Geometry check sheet. Reference: the model listing, model coordinates, mm. Round coordinates to 2 decimals unless told otherwise and drop trailing zeros. Loops run counter-clockwise (first coordinate to the right, second up) from the corner with the lowest first, then second, coordinate; pieces in that order, holes last. Notation, with made-up numbers: M 69,29 L 118,29 A19 cw 118,58 Z; hole C -14,82 d10. An arc over 180 degrees is marked long. Answer in a Markdown table with one row per item. Add a question column.
```python
from build123d import *

# Parameters (mm, degrees)
SKETCH1_R               = 8.89
SKETCH1_R_2             = 6.35
BOSS_EXTRUDE1_DEPTH     = 12.7
CUT_EXTRUDE1_DEPTH      = 29.341210278
CUT_EXTRUDE1_DEPTH_BACK = 29.341210278
SKETCH4_W               = 12.7
SKETCH4_H               = 5.08


# Read off the part's stored shape, not the designer's step: Revolve6
with BuildPart() as part:
    # Sketch1 → Boss-Extrude1 (new body)
    with BuildSketch(Plane(origin=(0, 0, 0), x_dir=(1, 0, 0), z_dir=(0, 1, 0))):
        with Locations(Location((0, 0, 0), (0, 0, 270))):
            Circle(SKETCH1_R)
        with Locations(Location((0, 0, 0), (0, 0, 270))):
            Circle(SKETCH1_R_2, mode=Mode.SUBTRACT)
    extrude(amount=BOSS_EXTRUDE1_DEPTH)

    # Revolve6 outline → Revolve6 (revolve)
    with BuildSketch(Plane.XY):
        Polygon((6.35, 0), (5.309918247, -2.54), (0, -17.711194992), (0, -25.4), (8.89, 0), align=None)
    revolve(axis=Axis((0, 0, 0), (0, 1, 0)))

    # Sketch4 → Cut-Extrude1 (cut, two sides: drawn at the far end of the back side and taken through both)
    with BuildSketch(Plane.XY.offset(-CUT_EXTRUDE1_DEPTH_BACK)):
        with Locations((0, -24.13)):
            Rectangle(SKETCH4_W, SKETCH4_H)
    extrude(amount=CUT_EXTRUDE1_DEPTH + CUT_EXTRUDE1_DEPTH_BACK, mode=Mode.SUBTRACT)


solid = part.part
```
1) Cross-section at A-A, the plane y = 10. Record the boundary of the cut face in (x, z).
2) Thickness scan on L1, parallel to Z at x = 0, y = 6.75; L2, parallel to Z at x = 2, y = 4. Record the ranges inside material, lowest first. Write a range as [from, to].
3) Draft check along Z on faces 1 (the flat face through (-6, 12.7, 4)), 2 (the conical face through (-3.432, -13.043, 2.632)), 3 (the cylindrical face through (-3.86, 6.26, -5.04)). Enter one of: +Z half, -Z half, draft (parallel to the pull), parting line (faces both ways), or undercut.
4) Go/stop test with flat-tipped pins: pin 1 (10 mm diameter, centred on x = -1, y = -16.5, fed in from -Z); pin 2 (5 mm diameter, centred on x = -3.5, y = -6.5, fed in from +Z). Record where each tip stops, or that it passes through.
5) Cross-section at B-B, the plane y = -15. Record the boundary of the cut face in (x, z).
Worked answers:
| question | item | result |
|---|---|---|
| 1 | outline | C 0,0 d17.78; hole C 0,0 d12.7 |
| 2 | L1 | z = [-8.89, -6.35], [6.35, 8.89] |
| 2 | L2 | z = [-8.66, -6.03], [6.03, 8.66] |
| 3 | face 1 | draft |
| 3 | face 2 | parting line |
| 3 | face 3 | undercut |
| 4 | pin 1 | stops at z = -4.84 |
| 4 | pin 2 | stops at z = 7.04 |
| 5 | outline | C 0,0 d7.28; hole C 0,0 d1.9 |
